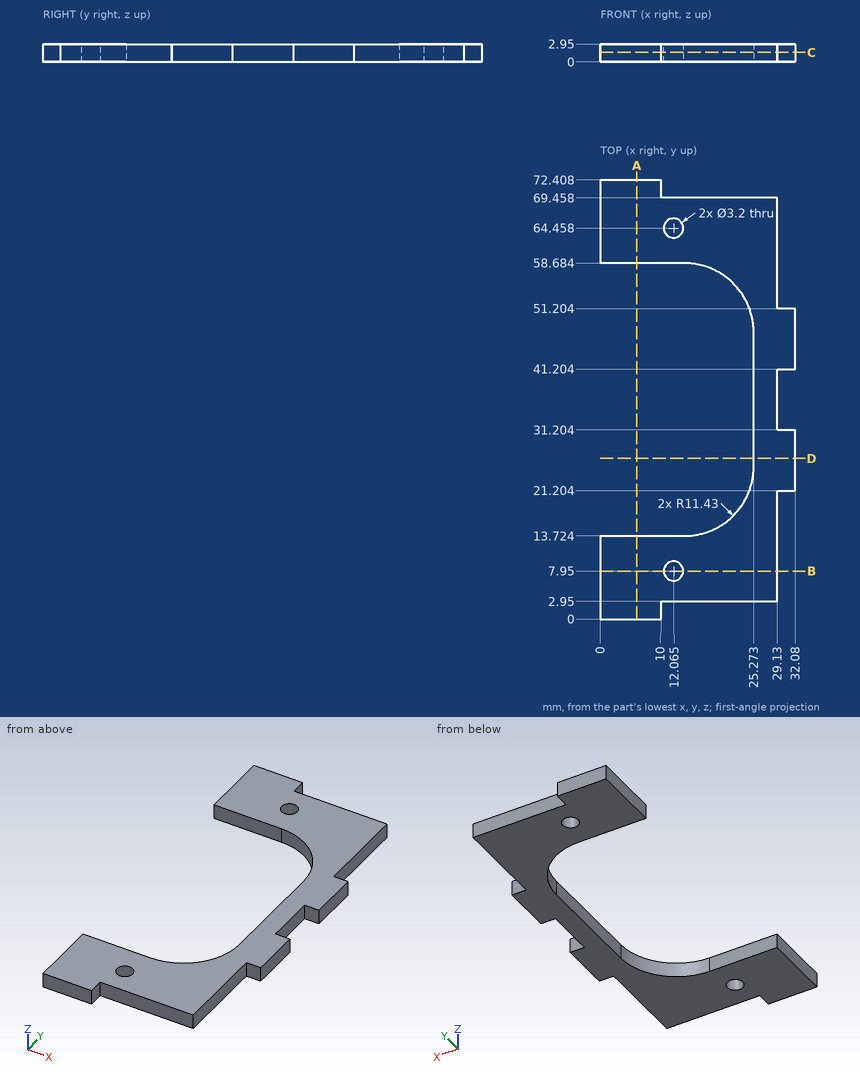
Answer from the drawing. Dimensions are ordinates in mm from the lowest x, y and z of the part. Coordinates: 2 decimals unless noted, no trailing zeros. Order: outer loops, then holes, each group sorted by start corner. A loop starts at its lowest first (then second) coordinate and runs counter-clockwise, first axis right, second up. Notation, with made-up numbers: (8.25, -33) - (21.25, -33) arc R24 ccw to (21.25, -15) - close; hole circle Ø1 at (85, 45). An arc over 180 degrees is marked (long way). Put each result on its own line as item: value. Start each with the question number.
1) Find section C-C (z = 1.55). State how many separate pieces and enclosed holes the cut face has, plus the area to 3 significant figures.
2) Find section D-D (y = 26.5). Give the vertices of the cut face in (x, z).
3) Flat-ended cylindrical pins translate along their axes: pin 1 (1.5 mm diameter, centred on x = 31, z = 1.5, fed in from +Y); pin 2 (1.5 mm diameter, centred on x = 19, z = 1.5, fed in from -Y); pin 3 (0.9 mm diameter, centred on y = 59.5, z = 1, fed in from +X). Find the tip coordinate at first contact, or state that the pin passes through.
4) Find the intervals of material crossed by line 1 (X direction, y = 7.95, z = 1.1) (3 decimals); line 2 (Y direction, x = 8, z = 1.7); line 3 (Y direction, x = 31, z = 2.55), in increasing order. Write a range as from..to.
5) Find section B-B (y = 7.95). Give the vertices of the cut face in (x, z) (3 decimals).
6) Find section A-A (x = 6). Give the vertices of the cut face in (y, z).
Results list:
1. separate pieces: 1
1. enclosed holes: 2
1. area: 959 mm^2
2. outline: (25.27, 0) - (32.08, 0) - (32.08, 2.95) - (25.27, 2.95) - close
3. pin 1: stops at y = 51.2
3. pin 2: stops at y = 2.95
3. pin 3: stops at x = 29.13
4. line 1: x = 0..10.465, 13.665..29.13
4. line 2: y = 0..13.72, 58.68..72.41
4. line 3: y = 21.2..31.2, 41.2..51.2
5. outline: (0, 0) - (10.465, 0) - (10.465, 2.95) - (0, 2.95) - close; (13.665, 0) - (29.13, 0) - (29.13, 2.95) - (13.665, 2.95) - close
6. outline: (0, 0) - (13.72, 0) - (13.72, 2.95) - (0, 2.95) - close; (58.68, 0) - (72.41, 0) - (72.41, 2.95) - (58.68, 2.95) - close
